CAD build for the part. Positions are in the model's coordinates, mm. Face numbers are marked on the shaded views. Coordinates: 2 decimals unless noted, no trailing zeros. Loops run counter-clockwise (first coordinate to the right, second up) from the corner with the lowest first, then second, coordinate; pieces in that order, holes last. Notation, with made-up numbers: (11.25, -28) -> (54.25, -28) arc R20 ccw to (54.25, -4) -> close; hole circle Ø7 at (-34.75, -9). An arc over 180 degrees is marked (long way). Return JSON: item names as keys, results as strings. Group by question number.
(1) Probe L1, parallel to Z at x = 0, y = -11.15; L2, parallel to Z at x = 1, y = -11; L3, parallel to Y at x = 25, z = 31. List the from-to ranges inside material, lowest first.
(2) Saw through at C-C on z = -21.59. Write the cut outline in (x, y).
(3) Mould opens along Z. For the marked faces 1, 2 and 3 say: pulls with the +Z half, pulls with the -Z half, needs draft (parallel to the pull), parting line crosses it, or undercut.
(4) Flat gauge pins, fed straight in: pin 1 Ø5 at (x, z) = (16, 36) entering from +Y; pin 2 Ø9 at (x, z) = (0, -21.59) entering from -Y; pin 3 Ø0.8 at (x, y) = (20, 0.5) entering from +Z; pin 4 Ø1.4 at (x, y) = (-10, -11) entering from +Z. Where does each tip first touch, or does it go through?
(5) Saw through at A-A on z = 31. Write the cut outline in (x, y).
(6) Saw through at D-D on x = 0. Write the cut outline in (y, z).
(7) Saw through at B-B on x = 23.5. Write the cut outline in (y, z), then the cut area to 3 significant figures.
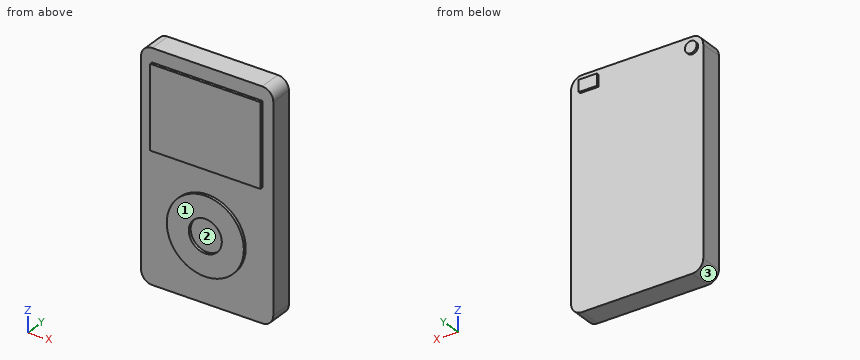
```python
from build123d import *

# Parameters (mm, degrees)
F1_DEPTH = 10.414
F2_W     = 50.8
F2_H     = 38.1
F2_R     = 17.78
F2_R_2   = 7.62
F3_DEPTH = 1.27
F4_R     = 2.69915
F4_W     = 8.422103
F4_H     = 5.414218
F5_DEPTH = 1.016


with BuildPart() as f1:
    # F0 (on Front) → F1 (new body)
    with BuildSketch(Plane.XZ):
        with BuildLine():
            ThreePointArc((30.48, 46.99), (28.992102, 50.582102), (25.4, 52.07))
            Line((25.4, 52.07), (-25.4, 52.07))
            ThreePointArc((-25.4, 52.07), (-28.992102, 50.582102), (-30.48, 46.99))
            Line((-30.48, 46.99), (-30.48, -46.99))
            ThreePointArc((-30.48, -46.99), (-28.992102, -50.582102), (-25.4, -52.07))
            Line((-25.4, -52.07), (25.4, -52.07))
            ThreePointArc((25.4, -52.07), (28.992102, -50.582102), (30.48, -46.99))
            Line((30.48, -46.99), (30.48, 46.99))
        make_face()
    extrude(amount=F1_DEPTH)

    # F2 (on face) → F3 (join)
    with BuildSketch(Plane.XZ.offset(10.414)):
        with Locations((0, 26.67)):
            Rectangle(F2_W, F2_H)
        with Locations((0, -21.59)):
            Circle(F2_R)
        with Locations((0, -21.59)):
            Circle(F2_R_2, mode=Mode.SUBTRACT)
    extrude(amount=F3_DEPTH)

    # F4 (on face) → F5 (join)
    with BuildSketch(Plane(origin=(0, 0, 0), x_dir=(-1, 0, 0), z_dir=(0, 1, 0))):
        with Locations((25.4, 46.99)):
            Circle(F4_R)
        with Locations((-22.108027, 47.073554)):
            Rectangle(F4_W, F4_H)
    extrude(amount=F5_DEPTH)


solid = f1.part
```
Geometry results:
{
 "1": {"L1": "-39.37 to -29.21, -13.97 to -3.81, 7.62 to 45.72", "L2": "-39.34 to -29.14, -14.04 to -3.84, 7.62 to 45.72", "L3": "-11.68 to 0"},
 "2": {"outline": "(-30.48, -10.41) -> (-17.78, -10.41) -> (-17.78, -11.68) -> (-7.62, -11.68) -> (-7.62, -10.41) -> (7.62, -10.41) -> (7.62, -11.68) -> (17.78, -11.68) -> (17.78, -10.41) -> (30.48, -10.41) -> (30.48, 0) -> (-30.48, 0) -> close"},
 "3": {"face 1": "needs draft", "face 2": "undercut", "face 3": "pulls with the -Z half"},
 "4": {"pin 1": "y = 0", "pin 2": "y = -10.41", "pin 3": "z = 49.78", "pin 4": "z = 52.07"},
 "5": {"outline": "(-30.48, -10.41) -> (-25.4, -10.41) -> (-25.4, -11.68) -> (25.4, -11.68) -> (25.4, -10.41) -> (30.48, -10.41) -> (30.48, 0) -> (-30.48, 0) -> close"},
 "6": {"outline": "(-11.68, -39.37) -> (-10.41, -39.37) -> (-10.41, -52.07) -> (0, -52.07) -> (0, 52.07) -> (-10.41, 52.07) -> (-10.41, 45.72) -> (-11.68, 45.72) -> (-11.68, 7.62) -> (-10.41, 7.62) -> (-10.41, -3.81) -> (-11.68, -3.81) -> (-11.68, -13.97) -> (-10.41, -13.97) -> (-10.41, -29.21) -> (-11.68, -29.21) -> close"},
 "7": {"outline": "(-11.68, 7.62) -> (-10.41, 7.62) -> (-10.41, -52.07) -> (0, -52.07) -> (0, 44.37) -> (1.02, 44.37) -> (1.02, 49.78) -> (0, 49.78) -> (0, 52.07) -> (-10.41, 52.07) -> (-10.41, 45.72) -> (-11.68, 45.72) -> close", "area": "1,140 mm²"}
}
